Geometry check sheet. Reference: drawing and pictorial views, mm from the part's lowest x, y, z. A direction names the side the tool comes from. Coordinates: 2 decimals unless noted, no trailing zeros. Loops run counter-clockwise (first coordinate to the right, second up) from the corner with the lowest first, then second, coordinate; pieces in that order, holes last. Notation, with made-up numbers: (23.25, 55.25) - (62.25, 55.25) arc R20 ccw to (62.25, 93.25) - close; hole circle Ø1 at (17.5, -19.75). An arc over 180 degrees is marked (long way). Use a Markdown table: item, result. Add a question column.
1) Draft check along X on the marked faces 1, 2, 3 and 4. Enter one of: pulls with the +X half, pulls with the -X half, needs draft (parallel to the pull), parting line crosses it, or undercut.
2) Thickness scan on line 1 (Z direction, x = 7, y = 88) (1 decimal); line 2 (X direction, y = 82, z = 18.5). Record the ranges inside material, lowest first.
3) Sectioned sample at B-B, the plane z = 101.6. Enter the section's corners in (x, y) (1 decimal).
4) Sectioned sample at C-C, the plane x = 64. Enter the section's corners in (y, z), then the cut area to 3 significant figures.
5) Sectioned sample at D-D, the plane x = 45. Enter the section's corners in (y, z).
6) Go/stop test with flat-tipped pins: P1, Ø6, axis at x = 69, z = 29.5, coming from the +Y side; P2, Ø1, axis at y = 70.5, z = 70, coming from the +X side; P3, Ø7.5, axis at x = 7.5, z = 106, coming from the -Y side (3 decimals). Record where each tip stops, or that it passes through.
7) Sectioned sample at A-A, the plane y = 88.9. Enter the section's corners in (x, z).
8) Tool access check on the marked faces 5 and 6. Record the directions out of +Z, -Z, +X, -X, +Y, -Y that give a thin tool (end or side, any length) a straight path to the whole face; none if there is none.
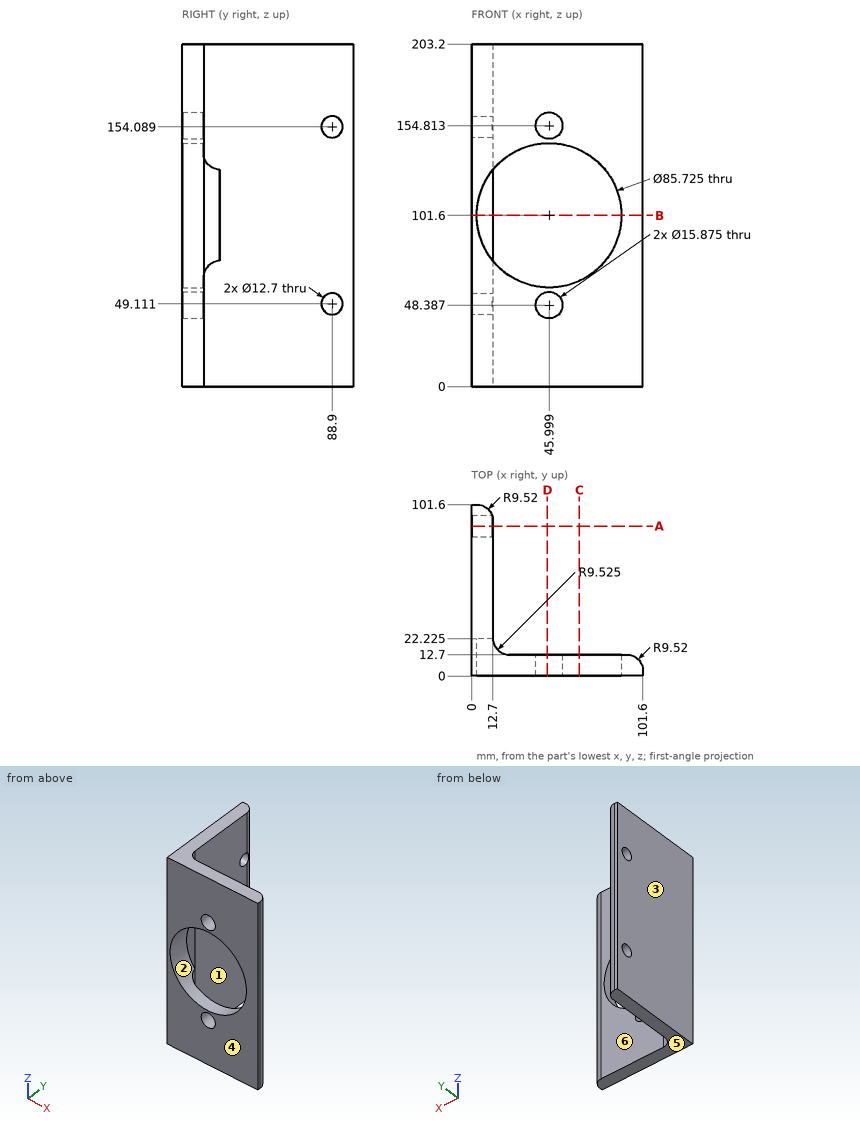
Solved:
| question | item | result |
|---|---|---|
| 1 | face 1 | pulls with the +X half |
| 1 | face 2 | undercut |
| 1 | face 3 | pulls with the -X half |
| 1 | face 4 | needs draft |
| 2 | line 1 | z = 0 to 42.8, 55.4 to 147.8, 160.4 to 203.2 |
| 2 | line 2 | x = 0 to 12.7 |
| 3 | outline | (0, 0) - (3.1, 0) - (3.1, 22.2) - (12.7, 22.2) - (12.7, 92.1) arc R9.5 ccw to (3.2, 101.6) - (0, 101.6) - close; (88.9, 0) - (101.6, 0) - (101.6, 3.2) arc R9.5 ccw to (92.1, 12.7) - (88.9, 12.7) - close |
| 4 | outline | (0, 0) - (12.7, 0) - (12.7, 62.7) - (0, 62.7) - close; (0, 140.5) - (12.7, 140.5) - (12.7, 203.2) - (0, 203.2) - close |
| 4 | area | 1,590 mm2 |
| 5 | outline | (0, 0) - (12.7, 0) - (12.7, 40.51) - (0, 40.51) - close; (0, 56.26) - (12.7, 56.26) - (12.7, 58.75) - (0, 58.75) - close; (0, 144.45) - (12.7, 144.45) - (12.7, 146.94) - (0, 146.94) - close; (0, 162.69) - (12.7, 162.69) - (12.7, 203.2) - (0, 203.2) - close |
| 6 | P1 | stops at y = 12.7 |
| 6 | P2 | stops at x = 12.7 |
| 6 | P3 | stops at y = 22.225 |
| 7 | outline | (0, 0) - (12.7, 0) - (12.7, 42.76) - (0, 42.76) - close; (0, 55.46) - (12.7, 55.46) - (12.7, 147.74) - (0, 147.74) - close; (0, 160.44) - (12.7, 160.44) - (12.7, 203.2) - (0, 203.2) - close |
| 8 | face 5 | -Z, +X, -X, +Y, -Y |
| 8 | face 6 | +Z, -Z, +X, +Y |
